```python
from build123d import *

# Parameters (mm, degrees)
F1_DEPTH      = 4
F3_DEPTH      = 65.001
F5_DEPTH      = 2
F8_DEPTH      = 20
F9_SIZE2      = 6.5817930688
F9_SIZE       = 3.8
F10_SIZE2     = 3.6397023427
F10_SIZE      = 10
F10_2_SIZE2   = 3.6397023427
F10_2_SIZE    = 10
F11_T1_DEPTH  = 19.0305228795
F11_T3_DEPTH  = 14.9081745177
F11_T5_DEPTH  = 30.6581745177
F11_T7_DEPTH  = 38.75
F11_T9_DEPTH  = 23
F11_T11_DEPTH = 28.25
F11_T13_DEPTH = 29
F11_T15_DEPTH = 25.3602976573
F11_T17_DEPTH = 15.6508497187


# Not quite as in the source:
# - a fillet or chamfer that OpenCascade refuses, or shapes differently, is made with other operations: its cross-section is extruded or revolved along the edge and cut away or added


with BuildPart() as f1:
    # F0 (on Top) → F1 (new body)
    with BuildSketch(Plane.XY):
        with BuildLine():
            Line((32.5, -20), (32.5, 20))
            Line((32.5, 20), (-32.5, 20))
            Line((-32.5, 20), (-32.5, -20))
            Line((-32.5, -20), (-22, -20))
            Line((-22, -20), (-22, 0))
            ThreePointArc((-22, 0), (-18.875, 3.125), (-15.75, 0))
            Line((-15.75, 0), (-15.75, -10))
            Line((-15.75, -10), (-10.75, -20))
            Line((-10.75, -20), (-5, -20))
            Line((-5, -20), (0, -10))
            Line((0, -10), (0, 0))
            ThreePointArc((0, 0), (3.125, 3.125), (6.25, 0))
            Line((6.25, 0), (6.25, -20))
            Line((6.25, -20), (32.5, -20))
        make_face()
    extrude(amount=F1_DEPTH)

    # F2 (on face) → F3 (cut, through all)
    with BuildSketch(Plane(origin=(-32.5, 0, 0), x_dir=(0, -1, 0), z_dir=(-1, 0, 0))):
        with BuildLine():
            Line((-1.25, 0), (1.25, 0))
            ThreePointArc((1.25, 0), (0, 1.25), (-1.25, 0))
        make_face()
    extrude(amount=-F3_DEPTH, mode=Mode.SUBTRACT)

    # F4 (on face) → F5 (join)
    with BuildSketch(Plane.XY):
        with BuildLine():
            ThreePointArc((0, 0), (0.0659177721, 0.6384676365), (0.2608901907, 1.25))
            Line((0.2608901907, 1.25), (-16.0108901907, 1.25))
            ThreePointArc((-16.0108901907, 1.25), (-15.8159177721, 0.6384676365), (-15.75, 0))
            Line((-15.75, 0), (-15.75, -1.25))
            Line((-15.75, -1.25), (0, -1.25))
            Line((0, -1.25), (0, 0))
        make_face()
    extrude(amount=F5_DEPTH)

    # F7 (on offset) → F8 (cut)
    with BuildSketch(Plane(origin=(-17.75, 0, 0), x_dir=(0, -1, 0), z_dir=(-1, 0, 0))):
        with BuildLine():
            Line((1.25, 4), (0, 4))
            Line((0, 4), (-1.25, 4))
            ThreePointArc((-1.25, 4), (0, 2.75), (1.25, 4))
        make_face()
    extrude(amount=-F8_DEPTH, mode=Mode.SUBTRACT)

    # F9
    f9_edges = [f1.edges().sort_by_distance(p)[0] for p in [
        (-7.875, -20, 4),
    ]]
    f9_side = f1.faces().sort_by_distance((-7.875, -20, 2))[0]
    chamfer(f9_edges, length=F9_SIZE, length2=F9_SIZE2, reference=f9_side)

    # F10
    f10_edges = [f1.edges().sort_by_distance(p)[0] for p in [
        (-27.25, -20, 0),
    ]]
    f10_side = f1.faces().sort_by_distance((-27.25, -10.625, 0))[0]
    chamfer(f10_edges, length=F10_SIZE, length2=F10_SIZE2, reference=f10_side)

    # F10#2
    f10_2_edges = [f1.edges().sort_by_distance(p)[0] for p in [
        (19.375, -20, 0),
    ]]
    f10_2_side = f1.faces().sort_by_distance((19.375, -10.625, 0))[0]
    chamfer(f10_2_edges, length=F10_2_SIZE, length2=F10_2_SIZE2, reference=f10_2_side)

    # F11: fillet of radius 5 on 14 edges, made by hand

    # F11_s2 → F11_t1 (cut)
    with BuildSketch(Plane.YZ.offset(-17.3902614398)):
        with BuildLine():
            ThreePointArc((-12.0784609691, 4), (-13.3725561946, 3.8296291314), (-14.5784609691, 3.3301270189))
            Line((-14.5784609691, 3.3301270189), (-13.4182069312, 4))
            Line((-13.4182069312, 4), (-12.0784609691, 4))
        make_face()
    extrude(amount=F11_T1_DEPTH, mode=Mode.SUBTRACT)

    # F11_s4 → F11_t3 (cut)
    with BuildSketch(Plane.YZ.offset(-34.7040872589)):
        with BuildLine():
            ThreePointArc((-9.1183650965, 0), (-9.9866059848, 0.0759612349), (-10.8284658131, 0.3015368961))
            Line((-10.8284658131, 0.3015368961), (-10, 0))
            Line((-10, 0), (-9.1183650965, 0))
        make_face()
    extrude(amount=F11_T3_DEPTH, mode=Mode.SUBTRACT)

    # F11_s6 → F11_t5 (cut)
    with BuildSketch(Plane.YZ.offset(4.0459127411)):
        with BuildLine():
            ThreePointArc((-9.1183650965, 0), (-9.9866059848, 0.0759612349), (-10.8284658131, 0.3015368961))
            Line((-10.8284658131, 0.3015368961), (-10, 0))
            Line((-10, 0), (-9.1183650965, 0))
        make_face()
    extrude(amount=F11_T5_DEPTH, mode=Mode.SUBTRACT)

    # F11_s8 → F11_t7 (cut)
    with BuildSketch(Plane.YZ):
        with BuildLine():
            ThreePointArc((-3.75, 0), (-2.1688611699, 0.2565835097), (-0.75, 1))
            ThreePointArc((-0.75, 1), (-1.1180339887, 0.5590169944), (-1.25, 0))
            Line((-1.25, 0), (-3.75, 0))
        make_face()
    extrude(amount=F11_T7_DEPTH, mode=Mode.SUBTRACT)

    # F11_s10 → F11_t9 (cut)
    with BuildSketch(Plane.YZ.offset(-38.75)):
        with BuildLine():
            ThreePointArc((-0.75, 1), (-2.1688611699, 0.2565835097), (-3.75, 0))
            Line((-3.75, 0), (-1.25, 0))
            ThreePointArc((-1.25, 0), (-1.1180339887, 0.5590169944), (-0.75, 1))
        make_face()
    extrude(amount=F11_T9_DEPTH, mode=Mode.SUBTRACT)

    # F11_s12 → F11_t11 (cut)
    with BuildSketch(Plane.YZ.offset(-22)):
        with BuildLine():
            ThreePointArc((-0.75, 3), (-2.1688611699, 3.7434164903), (-3.75, 4))
            Line((-3.75, 4), (-1.25, 4))
            ThreePointArc((-1.25, 4), (-1.1180339887, 3.4409830056), (-0.75, 3))
        make_face()
    extrude(amount=F11_T11_DEPTH, mode=Mode.SUBTRACT)

    # F11_s14 → F11_t13 (cut)
    with BuildSketch(Plane.XY.offset(-12.5)):
        with BuildLine():
            ThreePointArc((-27.5, 20), (-31.0355339059, 18.5355339059), (-32.5, 15))
            Line((-32.5, 15), (-32.5, 20))
            Line((-32.5, 20), (-27.5, 20))
        make_face()
        with BuildLine():
            ThreePointArc((32.5, 15), (31.0355339059, 18.5355339059), (27.5, 20))
            Line((27.5, 20), (32.5, 20))
            Line((32.5, 20), (32.5, 15))
        make_face()
    extrude(amount=F11_T13_DEPTH, mode=Mode.SUBTRACT)

    # F11_s16 → F11_t15 (cut)
    with BuildSketch(Plane.XY.offset(-8.8602976573)):
        with BuildLine():
            ThreePointArc((-32.5, -15), (-31.0355339059, -18.5355339059), (-27.5, -20))
            Line((-27.5, -20), (-32.5, -20))
            Line((-32.5, -20), (-32.5, -15))
        make_face()
        with BuildLine():
            ThreePointArc((-22, -15), (-23.4644660941, -18.5355339059), (-27, -20))
            Line((-27, -20), (-22, -20))
            Line((-22, -20), (-22, -15))
        make_face()
        with BuildLine():
            ThreePointArc((11.25, -20), (7.7144660941, -18.5355339059), (6.25, -15))
            Line((6.25, -15), (6.25, -20))
            Line((6.25, -20), (11.25, -20))
        make_face()
        with BuildLine():
            ThreePointArc((32.5, -15), (31.0355339059, -18.5355339059), (27.5, -20))
            Line((27.5, -20), (32.5, -20))
            Line((32.5, -20), (32.5, -15))
        make_face()
    extrude(amount=F11_T15_DEPTH, mode=Mode.SUBTRACT)

    # F11_s18 → F11_t17 (cut)
    with BuildSketch(Plane.XY.offset(-7.7254248594)):
        with BuildLine():
            ThreePointArc((-8.0901699437, -20), (-5.4615143832, -19.2532540418), (-3.6180339887, -17.2360679775))
            Line((-3.6180339887, -17.2360679775), (-5, -20))
            Line((-5, -20), (-8.0901699437, -20))
        make_face()
        with BuildLine():
            ThreePointArc((-12.1319660113, -17.2360679775), (-10.2884856168, -19.2532540418), (-7.6598300563, -20))
            Line((-7.6598300563, -20), (-10.75, -20))
            Line((-10.75, -20), (-12.1319660113, -17.2360679775))
        make_face()
    extrude(amount=F11_T17_DEPTH, mode=Mode.SUBTRACT)


solid = f1.part
```
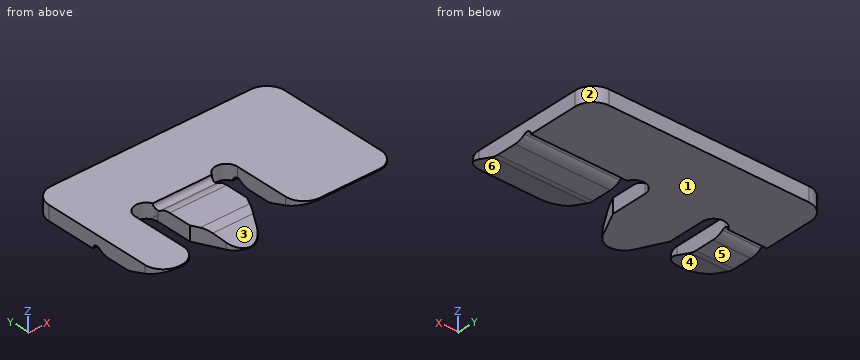
Work out the finished part from the listing and answer in its coordinate system (mm). Face numbers are marked on the shaded views. A direction names the side the tool comes from. Coordinates: 2 decimals unless noted, no trailing zeros. Loops run counter-clockwise (first coordinate to the right, second up) from the corner with the lowest first, then second, coordinate; pieces in that order, holes last. Notation, with made-up numbers: (57, 73.5) -> (90, 73.5) arc R23 ccw to (90, 92.5) -> close; hole circle Ø4 at (-7.5, 51). An arc over 180 degrees is marked (long way). Answer as CSV lines item,"result".
Q1. This flat-tipped pin is pushed along its axis until it touches: pin 1 (1 mm diameter, centred on x = -22.5, z = 2.5, fed in from -Y). Where does it stop, or does it pass through?
Findings:
pin 1,"stops at y = -17.81"
Q2. For a pull along X with two mould halves and no side action, classify the marked faces 1, 2 and 3 as +X half, -X half, draft (parallel to the pull), parting line (faces both ways), or undercut.
Findings:
face 1,"draft"
face 2,"+X half"
face 3,"undercut"
Q3. The part is cut by section B-B on x = 13.5. Write down the section's boundary in (y, z).
Findings:
outline,"(-20, 3.64) -> (-10.83, 0.3) arc R5 ccw to (-9.12, 0) -> (-3.75, 0) arc R5 ccw to (-0.75, 1) arc R1.25 cw to (1.25, 0) -> (20, 0) -> (20, 4) -> (-20, 4) -> close"
Q4. The part is cut by section C-C on x = -23. Write down the section's boundary in (y, z).
Findings:
outline,"(-18, 2.91) -> (-10.83, 0.3) arc R5 ccw to (-9.12, 0) -> (-3.75, 0) arc R5 ccw to (-0.75, 1) arc R1.25 cw to (1.25, 0) -> (20, 0) -> (20, 4) -> (-18, 4) -> close"
Q5. A tool of negligible diameter and unlimited length cuts with its end or side. For the marked faces 4, 5 and 6, from which of +Z, -Z, +X, -X, +Y, -Y can it reach the whole face along a straight path? Write none if from no direction.
Findings:
face 4,"-Z, -X, -Y"
face 5,"-Z, +X, -X, +Y, -Y"
face 6,"-Z, +X, -Y"
Q6. Find the intervals of material crossed by probe 1 along X at (y, z) = (-8, 3.7); probe 2 along Y at (x, z) = (4, 1.7); probe 3 along X at (y, z) = (-12, 2.9), in increasing order.
Findings:
probe 1,"x = -32.5 to -22, -15.75 to 0, 6.25 to 32.5"
probe 2,"y = 3 to 20"
probe 3,"x = -32.5 to -22, -14.75 to -1, 6.25 to 32.5"
Q7. The part is cut by section A-A on y = -6. Write down the section's boundary in (x, z), and give its area (3 significant figures).
Findings:
outline,"(-32.5, 0) -> (-22, 0) -> (-22, 4) -> (-32.5, 4) -> close; (-15.75, 0) -> (0, 0) -> (0, 4) -> (-15.75, 4) -> close; (6.25, 0) -> (32.5, 0) -> (32.5, 4) -> (6.25, 4) -> close"
area,"210 mm²"
